Verification items for the finished model (mm, model axes). Face numbers are marked on the shaded views. A direction names the side the tool comes from. Coordinates: 2 decimals unless noted, no trailing zeros. Order: outer loops, then holes, each group sorted by start corner. A loop starts at its lowest first (then second) coordinate and runs counter-clockwise, first axis right, second up. Notation, with made-up numbers: M -3.75,39 L 19.25,39 A36 ccw 19.25,73 Z; hole C 46,-39.5 d1. An arc over 180 degrees is marked long. Return JSON: item names as keys, results as strings. Group by question number.
1. Section check D-D, the plane z = 10. Record the cut outline in (x, y).
2. Gauge pin test, flat ends, axial feed: pin 1 (10 mm diameter, centred on y = 3, z = 17, fed in from -X); pin 2 (1.5 mm diameter, centred on y = 4, z = 31.5, fed in from -X); pin 3 (4 mm diameter, centred on x = 20.5, z = 7, fed in from +Y); pin 4 (6 mm diameter, centred on x = -22, y = -4, fed in from +Z). Record the tip position at first contact, or that the pin passes through.
3. Set-up check for the marked faces 1 and 2: record each of +Z, -Z, +X, -X, +Y, -Y from which the full face is reachable in a straight line by a thin tool's end or side.
4. Section check C-C, the plane y = 4.5. Record the cut outline in (x, z), plus the area to 3 significant figures.
5. Material ranges on line 1 along Z through (x, y) = (0, 2.5); line 2 along Y through (x, z) = (0, 31); line 3 along Y through (x, z) = (-39.5, 2.25), recorded low to high.
6. Section check B-B, the plane x = 0. Record the cut outline in (y, z), plus the area to 3 significant figures.
7. Section check A-A, the plane x = -39.5. Record the cut outline in (y, z).
```python
from build123d import *

# Parameters (mm, degrees)
CROQUIS1_R                 = 5.99
SALIENTE_EXTRUIR1_DEPTH    = 43.3
CROQUIS2_R                 = 1.75
CORTAR_EXTRUIR1_DEPTH      = 7.5
CROQUIS3_R                 = 45
SALIENTE_EXTRUIR2_DEPTH    = 3.2
CORTAR_EXTRUIR2_DEPTH      = 77.973307118
CORTAR_EXTRUIR2_DEPTH_BACK = 5
CROQUIS5_R                 = 2.15


with BuildPart() as part:
    # Croquis1 → Saliente-Extruir1 (new body)
    with BuildSketch(Plane.XY):
        with Locations(Location((0, 0, 0), (0, 0, 180))):
            Circle(CROQUIS1_R)
        with BuildLine():
            Line((-1.5, 1.322875656), (1.5, 1.322875656))
            ThreePointArc((1.5, 1.322875656), (0, -2), (-1.5, 1.322875656))
        make_face(mode=Mode.SUBTRACT)
    extrude(amount=SALIENTE_EXTRUIR1_DEPTH)

    # Croquis2 → Cortar-Extruir1 (cut)
    with BuildSketch(Plane(origin=(0, 1.322875656, 0), x_dir=(1, 0, 0), z_dir=(0, 1, 0))):
        with Locations((0, -40.05)):
            Circle(CROQUIS2_R)
        with Locations((0, -34.55)):
            Circle(CROQUIS2_R)
    extrude(amount=CORTAR_EXTRUIR1_DEPTH, mode=Mode.SUBTRACT)

    # Croquis3 → Saliente-Extruir2 (add)
    with BuildSketch(Plane(origin=(0, 0, 0), x_dir=(-1, 0, 0), z_dir=(0, 0, -1))):
        Circle(CROQUIS3_R)
    extrude(amount=-SALIENTE_EXTRUIR2_DEPTH)

    # Croquis5 → Cortar-Extruir2 (cut, two sides: drawn at the far end of the back side and taken through both)
    with BuildSketch(Plane(origin=(0, 0, 0), x_dir=(-1, 0, 0), z_dir=(0, 0, -1)).offset(-CORTAR_EXTRUIR2_DEPTH_BACK)):
        with Locations(Location((-39.5, 0, 0), (0, 0, 180))):
            Circle(CROQUIS5_R)
        with Locations(Location((39.5, 0, 0), (0, 0, 180))):
            Circle(CROQUIS5_R)
        Polygon((0, 10), (-75, 10), (-75, 50), (75, 50), (75, 10), align=None)
        Polygon((75, -50), (75, -10), (0, -10), (-75, -10), (-75, -50), align=None)
    extrude(amount=CORTAR_EXTRUIR2_DEPTH + CORTAR_EXTRUIR2_DEPTH_BACK, mode=Mode.SUBTRACT)


solid = part.part
```
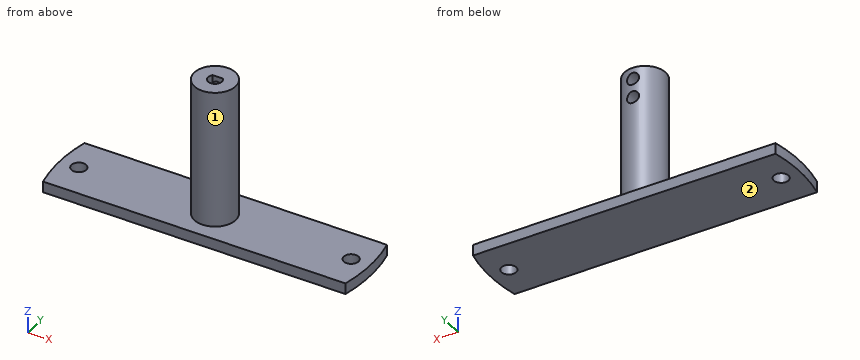
Answers follow:
{
 "1": {"outline": "C 0,0 d11.98; hole M -1.5,1.32 A2 ccw long 1.5,1.32 Z"},
 "2": {"pin 1": "x = -5.99", "pin 2": "x = -5.03", "pin 3": "through", "pin 4": "z = 3.2"},
 "3": {"face 1": "+Z", "face 2": "-Z, +X, -X, +Y, -Y"},
 "4": {"outline": "M -44.77,0 L 44.77,0 L 44.77,3.2 L 3.95,3.2 L 3.95,43.3 L -3.95,43.3 L -3.95,3.2 L -44.77,3.2 Z; hole C 0,34.55 d3.5; hole C 0,40.05 d3.5", "area": "584 mm^2"},
 "5": {"line 1": "0 to 32.8, 36.3 to 38.3, 41.8 to 43.3", "line 2": "-5.99 to -2, 1.32 to 5.99", "line 3": "-10 to -2.15, 2.15 to 10"},
 "6": {"outline": "M -10,0 L 10,0 L 10,3.2 L 5.99,3.2 L 5.99,32.8 L 1.32,32.8 L 1.32,3.2 L -2,3.2 L -2,43.3 L -5.99,43.3 L -5.99,3.2 L -10,3.2 Z; M 1.32,36.3 L 5.99,36.3 L 5.99,38.3 L 1.32,38.3 Z; M 1.32,41.8 L 5.99,41.8 L 5.99,43.3 L 1.32,43.3 Z", "area": "378 mm^2"},
 "7": {"outline": "M -10,0 L -2.15,0 L -2.15,3.2 L -10,3.2 Z; M 2.15,0 L 10,0 L 10,3.2 L 2.15,3.2 Z"}
}
